Part model, mm, in its own coordinate system. Face numbers are marked on the shaded views. A direction names the side the tool comes from. Round coordinates to 2 decimals unless told otherwise and drop trailing zeros. Order: outer loops, then holes, each group sorted by start corner. A loop starts at its lowest first (then second) coordinate and runs counter-clockwise, first axis right, second up. Notation, with made-up numbers: (28, 64) - (48, 64) arc R20 cw to (48, 88) - close; hole circle Ø2 at (-30.75, -9). An arc over 180 degrees is marked (long way). Return JSON: item names as keys, results as strings. Group by question number.
Item 1: Drop a flat-ended pin along its axis: pin 1 (3 mm diameter, centred on x = 4.5, y = -25, fed in from -Z). Give the stop position or say it passes through.
Item 2: Probe probe 1 along Y at (x, z) = (-2, 12); probe 2 along X at (y, z) = (-33, 14.5); probe 3 along X at (y, z) = (11.5, 5). List the from-to ranges inside material, lowest first.
Item 3: Saw through at B-B on y = 15. List the corners of the cut face in (x, z).
Item 4: Saw through at D-D on y = -33. List the corners of the cut face in (x, z), and give its area (3 significant figures).
Item 5: Saw through at C-C on z = 6. List the corners of the cut face in (x, y), and give its area (3 significant figures).
Item 6: Saw through at A-A on x = 0.5. List the corners of the cut face in (y, z).
Item 7: Two-plate mould, pull along X, no slides. Class the marked faces 1, 2, 3 and 4: released by +X, released by -X, zero draft, split by the parting line, or undercut.
Item 8: Tool access for the marked faces 5, 6 and 7: list every direction of +Z, -Z, +X, -X, +Y, -Y with a clear straight run to the whole face (end or side of a thin tool).
```python
from build123d import *

# Parameters (mm, degrees)
SKETCH3_W           = 53
SKETCH3_H           = 85
BOSS_EXTRUDE1_DEPTH = 20
SKETCH4_W           = 43
SKETCH4_H           = 75
CUT_EXTRUDE1_DEPTH  = 10
SKETCH5_W           = 26.321433762
SKETCH5_H           = 38.399655618
CUT_EXTRUDE2_DEPTH  = 10


with BuildPart() as part:
    # Sketch3 → Boss-Extrude1 (new body)
    with BuildSketch(Plane.XY):
        Rectangle(SKETCH3_W, SKETCH3_H)
    extrude(amount=BOSS_EXTRUDE1_DEPTH)

    # Sketch4 → Cut-Extrude1 (cut)
    with BuildSketch(Plane.XY.offset(20)):
        Rectangle(SKETCH4_W, SKETCH4_H)
    extrude(amount=-CUT_EXTRUDE1_DEPTH, mode=Mode.SUBTRACT)

    # Sketch5 → Cut-Extrude2 (cut)
    with BuildSketch(Plane(origin=(0, 0, 0), x_dir=(-1, 0, 0), z_dir=(0, 0, -1))):
        Rectangle(SKETCH5_W, SKETCH5_H)
    extrude(amount=-CUT_EXTRUDE2_DEPTH, mode=Mode.SUBTRACT)


solid = part.part
```
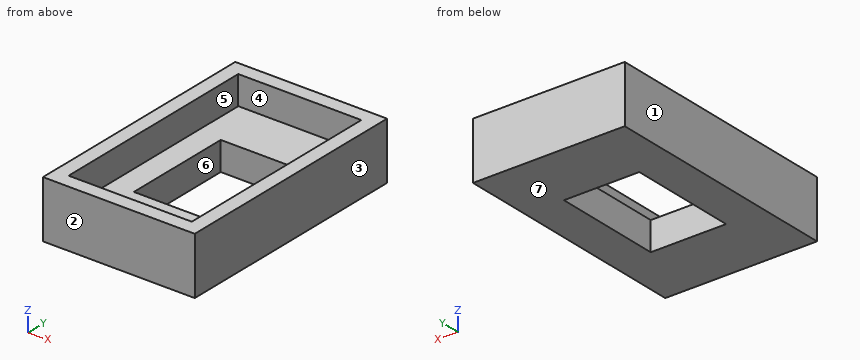
Filled in:
{
 "1": {"pin 1": "stops at z = 0"},
 "2": {"probe 1": "y = -42.5 to -37.5, 37.5 to 42.5", "probe 2": "x = -26.5 to -21.5, 21.5 to 26.5", "probe 3": "x = -26.5 to -13.16, 13.16 to 26.5"},
 "3": {"outline": "(-26.5, 0) - (-13.16, 0) - (-13.16, 10) - (-21.5, 10) - (-21.5, 20) - (-26.5, 20) - close; (13.16, 0) - (26.5, 0) - (26.5, 20) - (21.5, 20) - (21.5, 10) - (13.16, 10) - close"},
 "4": {"outline": "(-26.5, 0) - (26.5, 0) - (26.5, 20) - (21.5, 20) - (21.5, 10) - (-21.5, 10) - (-21.5, 20) - (-26.5, 20) - close", "area": "630 mm^2"},
 "5": {"outline": "(-26.5, -42.5) - (26.5, -42.5) - (26.5, 42.5) - (-26.5, 42.5) - close; hole (-13.16, -19.2) - (13.16, -19.2) - (13.16, 19.2) - (-13.16, 19.2) - close", "area": "3,490 mm^2"},
 "6": {"outline": "(-42.5, 0) - (-19.2, 0) - (-19.2, 10) - (-37.5, 10) - (-37.5, 20) - (-42.5, 20) - close; (19.2, 0) - (42.5, 0) - (42.5, 20) - (37.5, 20) - (37.5, 10) - (19.2, 10) - close"},
 "7": {"face 1": "released by -X", "face 2": "zero draft", "face 3": "released by +X", "face 4": "undercut"},
 "8": {"face 5": "+Z", "face 6": "+Z, -Z", "face 7": "-Z, +X, -X, +Y, -Y"}
}
